Part model, mm, in its own coordinate system. Give positions to 0.01 mm unless a question says otherwise; leave off trailing zeros. Order: outer loops, then holes, each group sorted by start corner. A loop starts at its lowest first (then second) coordinate and runs counter-clockwise, first axis right, second up. Notation, with made-up numbers: (28, -12.75) - (41, -12.75) arc R22 ccw to (41, 22.25) - close; hole circle Ø10 at (-30, 35). An arc over 180 degrees is marked (long way). Use a Markdown table: item, result. Add a question column.
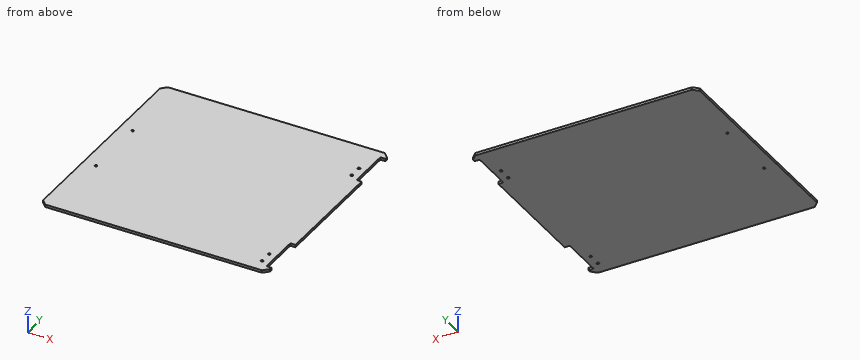
from build123d import *

# Parameters (mm, degrees)
SCHIZZO1_R                   = 2.5
SCHIZZO1_R_2                 = 2.499072061
SCHIZZO1_R_3                 = 2.25
ESTRUSIONE_ESTRUSIONE1_DEPTH = 5


with BuildPart() as part:
    # Schizzo1 → Estrusione-Estrusione1 (new body)
    with BuildSketch(Plane.XY):
        Polygon((-223, 204), (-213, 214), (213, 214), (223, 204), (223, 198.658355402), (213, 198.658355402), (213, 115.470714491), (223, 115.470714491), (223, -115.470714491), (213, -115.470714491), (213, -198.658355402), (223, -198.658355402), (223, -204), (213, -214), (-213, -214), (-223, -204), align=None)
        with Locations((198.51797805, 149.65244957)):
            Circle(SCHIZZO1_R, mode=Mode.SUBTRACT)
        with Locations((198.51797805, 124.65244957)):
            Circle(SCHIZZO1_R, mode=Mode.SUBTRACT)
        with Locations((198.494140307, -162.747561795)):
            Circle(SCHIZZO1_R_2, mode=Mode.SUBTRACT)
        with Locations((198.51797805, -187.74755043)):
            Circle(SCHIZZO1_R_2, mode=Mode.SUBTRACT)
        with Locations((-198, 64)):
            Circle(SCHIZZO1_R_3, mode=Mode.SUBTRACT)
        with Locations(Location((-198, -64, 0), (0, 0, 180))):
            Circle(SCHIZZO1_R_3, mode=Mode.SUBTRACT)
    extrude(amount=ESTRUSIONE_ESTRUSIONE1_DEPTH)


solid = part.part
1. Cut at A-A (y = -173.5). Write the cut outline in (x, z).
2. Drill centre lines: probe 1 along Y at (x, z) = (-198, 2.05); probe 2 along Y at (x, z) = (-200, 4.4); probe 3 along X at (y, z) = (-64, 3.15). Where is each one in solid material? Low to high. Write a range as [from, to].
3. Pin check, flat tips, straight feed: P1, Ø1.5, axis at x = 218.5, z = 1.5, coming from the -Y side; P2, Ø6.5, axis at x = 198.52, y = 149.65, coming from the -Z side; P3, Ø2.5, axis at y = 176.5, z = 2, coming from the +X side. Stop position of each tip, or through.
Responses:
| question | item | result |
|---|---|---|
| 1 | outline | (-223, 0) - (213, 0) - (213, 5) - (-223, 5) - close |
| 2 | probe 1 | y = [-214, -66.25], [-61.75, 61.75], [66.25, 214] |
| 2 | probe 2 | y = [-214, -65.03], [-62.97, 62.97], [65.03, 214] |
| 2 | probe 3 | x = [-223, -200.25], [-195.75, 223] |
| 3 | P1 | stops at y = -209.25 |
| 3 | P2 | stops at z = 0 |
| 3 | P3 | stops at x = 213 |
